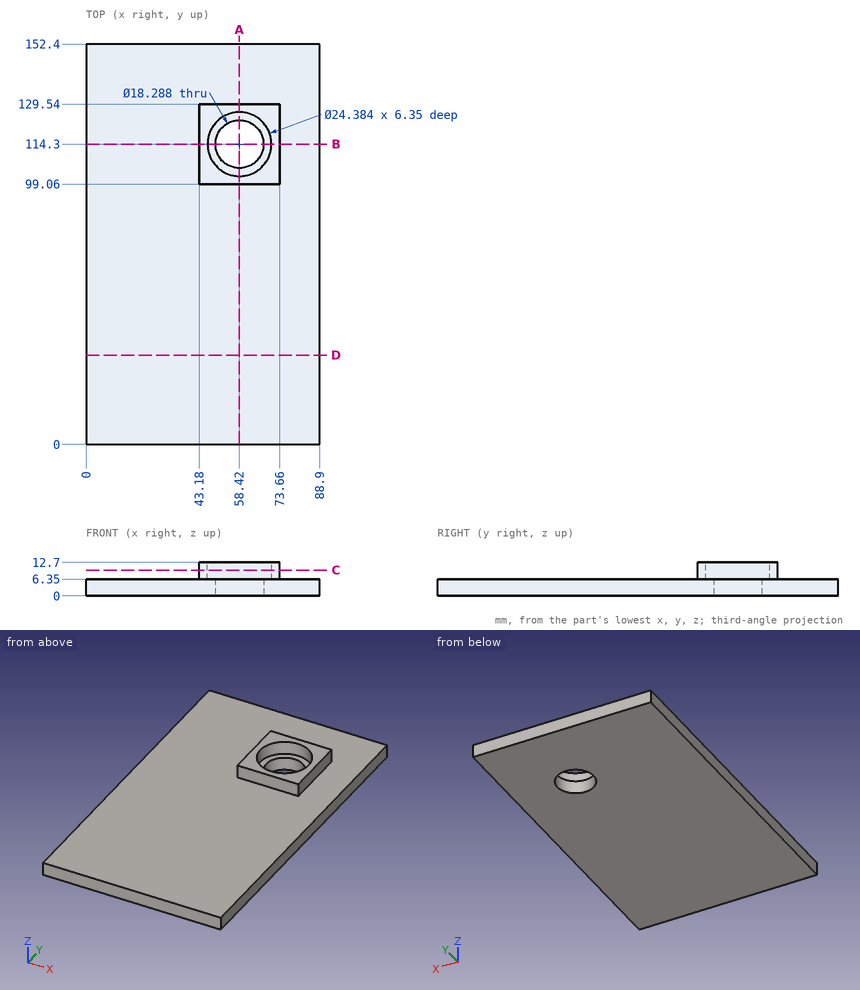
Geometry check sheet. Reference: drawing and pictorial views, mm from the part's lowest x, y, z. Round coordinates to 2 decimals unless told otherwise and drop trailing zeros. Write each loop counter-clockwise with the first axis right and the second up, starting at its lowest first coordinate (ties: lowest second). Pieces come first, ordered by that corner, then holes. Notation, with made-up numbers: (40, -3) -> (85, -3) arc R23 cw to (85, 32) -> close; hole circle Ø10 at (31, 9.25). An arc over 180 degrees is marked (long way). Put each result on its own line as item: value.
1) Cross-section at A-A, the plane x = 58.42. Enter the section's corners in (y, z).
Recorded:
outline: (0, 0) -> (105.16, 0) -> (105.16, 6.35) -> (102.11, 6.35) -> (102.11, 12.7) -> (99.06, 12.7) -> (99.06, 6.35) -> (0, 6.35) -> close; (123.44, 0) -> (152.4, 0) -> (152.4, 6.35) -> (129.54, 6.35) -> (129.54, 12.7) -> (126.49, 12.7) -> (126.49, 6.35) -> (123.44, 6.35) -> close
2) Depth check by flat-ended pin: P1, Ø3, axis at y = 109, z = 8, coming from the +X side; P2, Ø1, axis at x = 24, z = 7.5, coming from the -Y side; P3, Ø8, axis at x = 32.5, y = 135, coming from the +Z side; P4, Ø7, axis at x = 51.5, z = 9, coming from the -Y side. Enter the tip coordinate at first touch or a pass-through.
Recorded:
P1: stops at x = 73.66
P2: passes through
P3: stops at z = 6.35
P4: stops at y = 0
3) Thickness scan on probe 1 along Y at (x, z) = (58.42, 11); probe 2 along Y at (x, z) = (58.42, 2); probe 3 along Z at (x, y) = (50, 30). Record the ranges inside material, lowest first. Write a range as from..to.
Recorded:
probe 1: y = 99.06..102.11, 126.49..129.54
probe 2: y = 0..105.16, 123.44..152.4
probe 3: z = 0..6.35
4) Cross-section at B-B, the plane y = 114.3. Enter the section's corners in (x, z), plus the area to 3 significant figures.
Recorded:
outline: (0, 0) -> (49.28, 0) -> (49.28, 6.35) -> (46.23, 6.35) -> (46.23, 12.7) -> (43.18, 12.7) -> (43.18, 6.35) -> (0, 6.35) -> close; (67.56, 0) -> (88.9, 0) -> (88.9, 6.35) -> (73.66, 6.35) -> (73.66, 12.7) -> (70.61, 12.7) -> (70.61, 6.35) -> (67.56, 6.35) -> close
area: 487 mm2
5) Cross-section at D-D, the plane y = 34. Enter the section's corners in (x, z), plus the area to 3 significant figures.
Recorded:
outline: (0, 0) -> (88.9, 0) -> (88.9, 6.35) -> (0, 6.35) -> close
area: 565 mm2
6) Cross-section at C-C, the plane z = 9.75. Enter the section's corners in (x, y).
Recorded:
outline: (43.18, 99.06) -> (73.66, 99.06) -> (73.66, 129.54) -> (43.18, 129.54) -> close; hole circle Ø24.38 at (58.42, 114.3)
